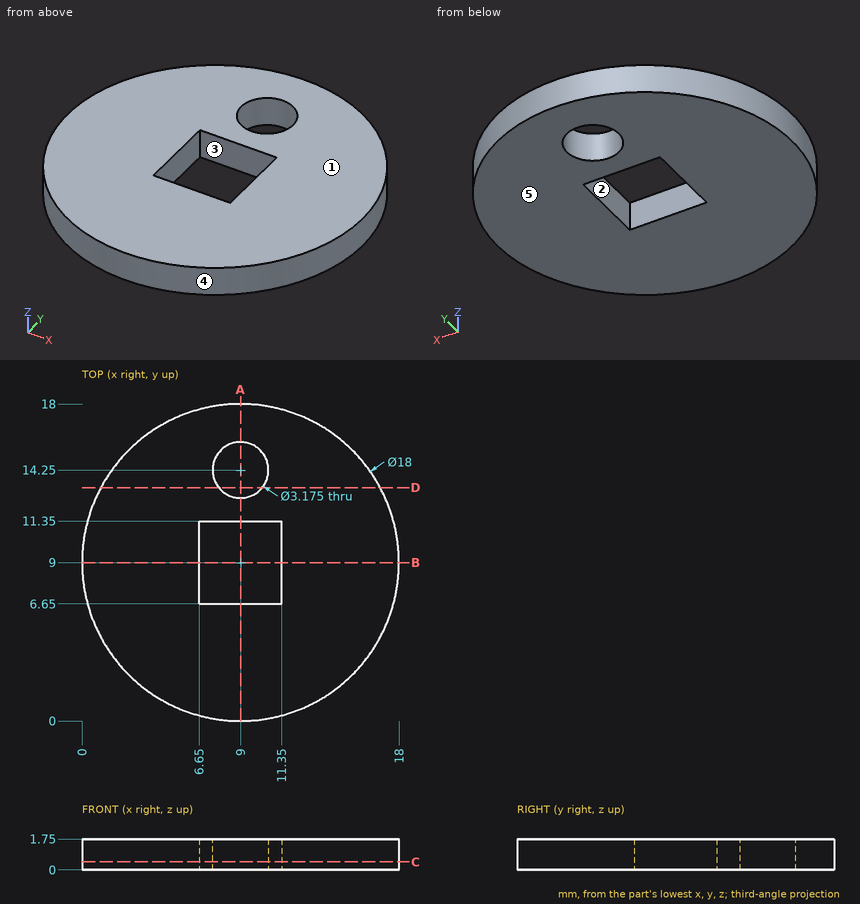
Geometry: see drawing. Coordinates: mm, zero at the bounding-box minimum. A direction names the side the tool comes from. Round coordinates to 2 decimals unless told otherwise and drop trailing zeros. Loops run counter-clockwise (first coordinate to the right, second up) from the corner with the lowest first, then second, coordinate; pieces in that order, holes last. Notation, with made-up numbers: (-13.5, -9.75) -> (4.5, -9.75) arc R27 ccw to (4.5, 26.25) -> close; hole circle Ø3 at (-29, 81.5). An arc over 180 degrees is marked (long way). Write each question's results on one line, items separated by ' | '.
1. Section A-A (x = 9). Return loops of the section in (y, z), and give its area (3 significant figures).
Geometry results:
outline: (0, 0) -> (6.65, 0) -> (6.65, 1.75) -> (0, 1.75) -> close; (11.35, 0) -> (12.66, 0) -> (12.66, 1.75) -> (11.35, 1.75) -> close; (15.84, 0) -> (18, 0) -> (18, 1.75) -> (15.84, 1.75) -> close | area: 17.7 mm2
2. Section B-B (y = 9). Return loops of the section in (x, z).
Geometry results:
outline: (0, 0) -> (6.65, 0) -> (6.65, 1.75) -> (0, 1.75) -> close; (11.35, 0) -> (18, 0) -> (18, 1.75) -> (11.35, 1.75) -> close
3. Set-up query: the marked faces 1 and 2. Return all of +Z, -Z, +X, -X, +Y, -Y with unobstructed straight access to the full face (end or side cutting, diameter ignored); none if empty.
Geometry results:
face 1: +Z, +X, -X, +Y, -Y | face 2: +Z, -Z
4. Section C-C (z = 0.45). State how many separate pieces and enclosed holes the cut face has, and give its area (3 significant figures).
Geometry results:
separate pieces: 1 | enclosed holes: 2 | area: 224 mm2
5. First-contact query: P1, Ø0.9, axis at x = 8.5, z = 1, coming from the +Y side; P2, Ø1, axis at y = 14.5, z = 0.5, coming from the +X side. Flat tips, straight axial feed; report the tip coordinate or a pass-through.
Geometry results:
P1: y = 18 | P2: x = 16.48
6. Mould query, pull axis Y, two halves, no side actions, for the marked faces 3, 4 and 5. Classes: +Y half, -Y half, draft (parallel to the pull), parting line (faces both ways), or undercut.
Geometry results:
face 3: undercut | face 4: parting line | face 5: draft
7. Ray query, line 1 (Y direction, x = 9, z = 0.45); line 2 (X direction, y = 9.25, z = 0.15); line 3 (X direction, y = 6.5, z = 0.65). Return the intervals inside material, ascending. Write a range as from..to.
Geometry results:
line 1: 0..6.65, 11.35..12.66, 15.84..18 | line 2: 0..6.65, 11.35..18 | line 3: 0.35..17.65
8. Section D-D (y = 13.25). Return loops of the section in (x, z).
Geometry results:
outline: (1.07, 0) -> (7.77, 0) -> (7.77, 1.75) -> (1.07, 1.75) -> close; (10.23, 0) -> (16.93, 0) -> (16.93, 1.75) -> (10.23, 1.75) -> close
